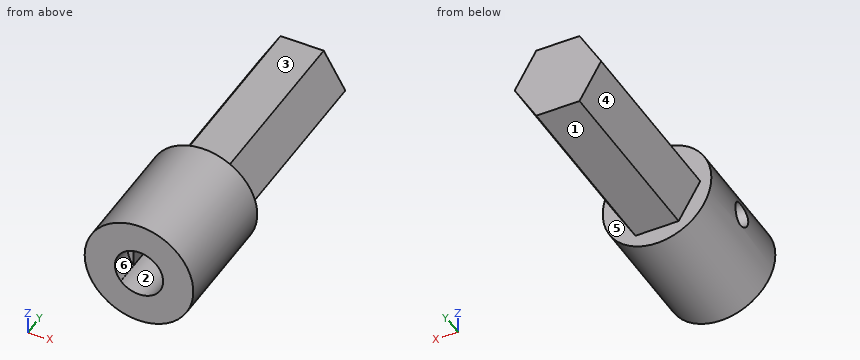
Autodesk Inventor part; units mm, degrees
ref_plane "YZ Plane" through (0, 0, 0) normal (1, 0, 0) x (0, 1, 0)
ref_plane "XZ Plane" through (0, 0, 0) normal (0, 1, 0) x (-1, 0, 0)
ref_plane "XY Plane" through (0, 0, 0) normal (0, 0, 1) x (1, 0, 0)
sketch "Sketch4" plane through (0, 0, 0) normal (0, 1, 0) x (-1, 0, 0)
  circle A0 centre (0, 0) radius 4.5
  dimension "d6" = 9
extrude "Extrusion2" add sketch "Sketch4" along normal blind 10
sketch "Sketch5" plane through (0, 10, 0) normal (0, 1, 0) x (1, 0, 0)
  circle A0 centre (0, 0) radius 2
  line L0 (-1.5, -1.3229) -> (-1.5, 1.3229)
  dimension "d9" = 4
  dimension "d10" = 3.5
extrude "Extrusion3" cut sketch "Sketch5" against normal blind 10 contours A0 L0 picked at (-0.1695, 0.3101)
sketch "Sketch6" plane through (0, 0, 0) normal (0, -1, 0) x (1, 0, 0)
  circle A0 centre (0, 0) radius 1.9934
extrude "Extrusion4" cut sketch "Sketch6" against normal blind 2
sketch "Sketch7" plane through (0, 10, 0) normal (0, 1, 0) x (1, 0, 0)
  line L0 (-3.58, 0) -> (-1.79, 3.1004)
  line L1 (-1.79, 3.1004) -> (1.79, 3.1004)
  line L2 (1.79, 3.1004) -> (3.58, 0)
  line L3 (3.58, 0) -> (1.79, -3.1004)
  line L4 (1.79, -3.1004) -> (-1.79, -3.1004)
  line L5 (-1.79, -3.1004) -> (-3.58, 0)
  point P0 (0, 0)
  point P1 (0, 0)
  dimension "d15" = 7.16
extrude "Extrusion5" add sketch "Sketch7" along normal blind 15.5 and the other way blind 0.75
sketch "Sketch14" plane through (-1.5, 0, 1.3129) normal (1, 0, 0) x (0, 0, -1)
  circle A0 centre (1.3129, 5.2313) radius 1
  point P0 (1.3129, 0)
  dimension "d38" = 2
extrude "Extrusion10" cut sketch "Sketch14" against normal blind 4
sketch "Sketch9" plane through (-1.5, 0, 1.3129) normal (1, 0, 0) x (0, 0, -1)
  circle A0 centre (1.3129, 5.7735) radius 1
  point P0 (1.3129, 0)
  dimension "d21" = 2
sketch "Sketch10" plane through (-3.75, 5.7735, 0) normal (-1, 0, 0) x (0, 0, 1)
  point P0 (0, -5.7735)
  point P1 (-0.001, 0.0019)
sketch "Sketch1" plane through (0, 0, 0) normal (0, 1, 0) x (-1, 0, 0)
  circle A0 centre (0, 0) radius 12.5
  dimension "d0" = 25
  dimension "d3" = 4
  dimension "d4" = 7
  dimension "d5" = 3.5
properties part number "As JGA To Mecanum_3DPrint"
The model under review builds one solid part; all positions refer to its coordinate system, in mm. Face numbers are marked on the shaded views. A direction names the side the tool comes from. Give positions to 0.01 mm unless a question says otherwise; leave off trailing zeros. Write each loop counter-clockwise with the first axis right and the second up, starting at its lowest first coordinate (ties: lowest second). Pieces come first, ordered by that corner, then holes.
1. For P1, Ø4, axis at y = 15.5, z = -2.5, coming from the +X side; P2, Ø5, axis at x = -2.5, y = 22, coming from the -Z side; P3, Ø3, axis at y = 3, z = 1, coming from the -X side; P4, Ø1, axis at x = 0.5, z = 0.5, coming from the -Y side, all flat-tipped, find the tip position at first contact; note any pin that passes through.
2. Tool access review of the marked faces 1, 2 and 3: name each direction out of +Z, -Z, +X, -X, +Y, -Y from which nothing blocks a thin tool from reaching the whole face with its end or side.
3. Add section C-C, the plane z = -2.25. Write out the cut boundary in (x, y).
4. Add section D-D, the plane y = 13.5. Write out the cut boundary in (x, z).
5. Add section A-A, the plane x = 0. Write out the cut boundary in (y, z), plus the area to 3 significant figures.
6. Add section B-B, the plane z = -0.5. Write out the cut boundary in (x, y), plus the area to 3 significant figures.
7. Wall thickness on L1, parallel to Y at x = -3, z = 0; L2, parallel to Z at x = 0, y = 5; L3, parallel to Y at x = 1.75, z = 3.25: over which ranges is each line inside the solid? List them lowest first.
8. Draft analysis for pull direction X (two halves, no side actions). For the marked faces 4, 5 and 6, state which applies: +X half, -X half, draft (parallel to the pull), parting line (faces both ways), or undercut.
Worked answers:
1. P1: stops at x = 3.29
1. P2: stops at z = -3.1
1. P3: stops at x = -4.5
1. P4: stops at y = 9.25
2. face 1: -Z, +X, -X, +Y
2. face 2: -Y
2. face 3: +Z, +X, -X, +Y
3. outline: (-3.9, 0) - (3.9, 0) - (3.9, 10) - (2.28, 10) - (2.28, 25.5) - (-2.28, 25.5) - (-2.28, 10) - (-3.9, 10) - close
4. outline: (-3.58, 0) - (-1.79, -3.1) - (1.79, -3.1) - (3.58, 0) - (1.79, 3.1) - (-1.79, 3.1) - close
5. outline: (0, -4.5) - (10, -4.5) - (10, -3.1) - (25.5, -3.1) - (25.5, 3.1) - (10, 3.1) - (10, 4.5) - (0, 4.5) - (0, 2) - (9.25, 2) - (9.25, -2) - (0, -2) - close
5. area: 149 mm2
6. outline: (-4.47, 0) - (-1.93, 0) - (-1.93, 2) - (-1.5, 2) - (-1.5, 4.37) - (-4.47, 4.37) - close; (-4.47, 6.1) - (-1.5, 6.1) - (-1.5, 9.25) - (1.94, 9.25) - (1.94, 0) - (4.47, 0) - (4.47, 10) - (3.29, 10) - (3.29, 25.5) - (-3.29, 25.5) - (-3.29, 10) - (-4.47, 10) - close
6. area: 154 mm2
7. L1: y = 0 to 4.23, 6.23 to 25.5
7. L2: z = -4.5 to -2, 2 to 4.5
7. L3: y = 0 to 10
8. face 4: -X half
8. face 5: draft
8. face 6: undercut
